Geometry check sheet. Reference: the model listing, model coordinates, mm. A direction names the side the tool comes from. Round coordinates to 2 decimals unless told otherwise and drop trailing zeros. Order: outer loops, then holes, each group sorted by start corner. A loop starts at its lowest first (then second) coordinate and runs counter-clockwise, first axis right, second up. Notation, with made-up numbers: M 39,-11 L 63,-11 A8 cw 63,-2 Z; hole C -16,-12 d5. An arc over 180 degrees is marked long. Answer as a JSON object with one key per item and string values. Group by question number.
```python
from build123d import *

# Parameters (mm, degrees)
CHAMFER1_SIZE      = 1
SKETCH2_R          = 1.1
CUT_EXTRUDE1_DEPTH = 31.813957876
CHAMFER2_SIZE      = 1


with BuildPart() as part:
    # Sketch1 → Revolve1 (revolve)
    with BuildSketch(Plane(origin=(0, 0, 0), x_dir=(0, 0, -1), z_dir=(1, 0, 0)), mode=Mode.PRIVATE) as revolve1_sk:
        Polygon((0, 21.5), (2, 21.5), (2, 20), (5, 20), (5, 13.6), (2, 13.6), (2, 12), (0, 12), align=None)
    revolve(revolve1_sk.sketch.rotate(Axis((0, 0, 0), (0, 0, -1)), 180), axis=Axis((0, 0, 0), (0, 0, -1)))

    # Chamfer1
    chamfer1_edges = [part.edges().sort_by_distance(p)[0] for p in [
        (0, 20, -5),
    ]]
    chamfer(chamfer1_edges, length=CHAMFER1_SIZE)

    # Sketch2 → Cut-Extrude1 (cut, through all)
    with BuildSketch(Plane(origin=(0, 0, -5), x_dir=(-1, 0, 0), z_dir=(0, 0, -1))):
        with Locations((12.990381057, -7.5)):
            Circle(SKETCH2_R)
        with Locations((-12.990381057, -7.5)):
            Circle(SKETCH2_R)
        with Locations(Location((0, 15, 0), (0, 0, 90))):
            Circle(SKETCH2_R)
    extrude(amount=-CUT_EXTRUDE1_DEPTH, mode=Mode.SUBTRACT)

    # Chamfer2
    chamfer2_edges = [part.edges().sort_by_distance(p)[0] for p in [
        (-11.890381057, -7.5, 0),
        (14.090381057, -7.5, 0),
        (0, 13.9, 0),
    ]]
    chamfer(chamfer2_edges, length=CHAMFER2_SIZE)


solid = part.part
```
1) Release check for a two-part mould opening along Y. For faces 1 (the flat face through (13, -16, -2)), 2 (the flat face through (10, -7, -2)), 3 (the cylindrical face through (-21.317, 2.799, -1.014)) record: +Y half, -Y half, draft (parallel to the pull), parting line (faces both ways), or undercut.
2) Sectioned sample at A-A (x = 0). Record the boundary of the cut face in (y, z).
3) Sectioned sample at D-D (y = -7.5). Count the separate pieces of the cut face and the enclosed holes in it, then the cut area to 3 significant figures.
4) Go/stop test with flat-tipped pins: P1, Ø1, axis at y = 7, z = -4.5, coming from the +X side; P2, Ø2.5, axis at x = -12.99, y = -7.5, coming from the +Z side; P3, Ø2, axis at y = 5.5, z = -4, coming from the +X side. Record where each tip stops, or that it passes through.
5) Sectioned sample at B-B (y = 0). Record the boundary of the cut face in (x, z), then the cut area to 3 significant figures.
6) Thickness scan on line 1 along Y through (x, z) = (1, -1.45); line 2 along Y through (x, z) = (1, -3.8); line 3 along X through (y, z) = (10, -1.2). Record the ranges inside material, lowest first. Write a range as [from, to].
7) Set-up check for faces 4 (the flat face through (10, -10, -5)), 5 (the cylindrical face through (-0.88, 19.98, -3.01)): record each of +Z, -Z, +X, -X, +Y, -Y from which the full face is reachable in a straight line by a thin tool's end or side.
8) Sectioned sample at C-C (z = -3.35). Record the boundary of the cut face in (x, y).
Final values:
{
 "1": {"face 1": "draft", "face 2": "undercut", "face 3": "parting line"},
 "2": {"outline": "M -21.5,-2 L -20,-2 L -20,-4 L -19,-5 L -13.6,-5 L -13.6,-2 L -12,-2 L -12,0 L -21.5,0 Z; M 12,-2 L 13.6,-2 L 13.6,-5 L 13.9,-5 L 13.9,-1 L 12.9,0 L 12,0 Z; M 16.1,-5 L 19,-5 L 20,-4 L 20,-2 L 21.5,-2 L 21.5,0 L 17.1,0 L 16.1,-1 Z"},
 "3": {"separate pieces": "4", "enclosed holes": "0", "area": "61.2 mm^2"},
 "4": {"P1": "stops at x = 18.77", "P2": "stops at z = -0.85", "P3": "stops at x = 19.49"},
 "5": {"outline": "M -21.5,-2 L -20,-2 L -20,-4 L -19,-5 L -13.6,-5 L -13.6,-2 L -12,-2 L -12,0 L -21.5,0 Z; M 12,-2 L 13.6,-2 L 13.6,-5 L 19,-5 L 20,-4 L 20,-2 L 21.5,-2 L 21.5,0 L 12,0 Z", "area": "75.4 mm^2"},
 "6": {"line 1": "y = [-21.48, -11.96], [11.96, 14.54], [15.46, 21.48]", "line 2": "y = [-19.97, -13.56], [13.56, 14.54], [15.46, 19.97]", "line 3": "x = [-19.03, -6.63], [6.63, 19.03]"},
 "7": {"face 4": "-Z, +X, -X, +Y, -Y", "face 5": "-Z"},
 "8": {"outline": "C 0,0 d40; hole C -12.99,-7.5 d2.2; hole C 0,0 d27.2; hole C 0,15 d2.2; hole C 12.99,-7.5 d2.2"}
}
